The listing builds one solid part. Answer for the finished solid, in the listing's coordinates (mm). A direction names the side the tool comes from. Coordinates: 2 decimals unless noted, no trailing zeros. Loops run counter-clockwise (first coordinate to the right, second up) from the corner with the lowest first, then second, coordinate; pieces in that order, holes last. Notation, with made-up numbers: M 44,2.5 L 72,2.5 A8 ccw 72,8.5 Z; hole C 28,-29.75 d1. An arc over 180 degrees is marked long. Answer as a JSON object with one key per item and string values. Group by question number.
1. A cutting plane is placed at B-B on x = 8.5. Give the vertices of the cut face in (y, z).
2. Given pin 1 (6 mm diameter, centred on x = 1, y = -4.5, fed in from -Z); pin 2 (0.6 mm diameter, centred on y = -6.5, z = 1, fed in from +X); pin 3 (0.6 mm diameter, centred on x = -4.5, z = 1.5, fed in from -Y), each flat-ended and moving along its own axis, determine where each tip first touches the part or whether it passes through.
3. Straight lines are drawn through the part: L1, parallel to X at y = -7, z = 0.5; L2, parallel to Y at x = -4.5, z = 1.3; L3, parallel to X at y = 4.5, z = 1.05. For each, find the intervals that lie inside material, in ascending order.
4. For faces 1 (the face through (-4, -4, 1)), 2 (the face through (8, -4, 1)), 3 (the face through (2, 0, 0)), determine the directions among +Z, -Z, +X, -X, +Y, -Y from which every point of the face is accessible in a straight line to the end or side of a thin tool.
5. A cutting plane is placed at C-C on y = 5. Give the vertices of the cut face in (x, z).
6. A cutting plane is placed at A-A on z = 0.8. Give the vertices of the cut face in (x, y), and give its area (3 significant figures).
from build123d import *

# Parameters (mm, degrees)
BOSS_EXTRUDE1_DEPTH = 2


with BuildPart() as part:
    # Sketch1 → Boss-Extrude1 (new body)
    with BuildSketch(Plane.XY):
        with BuildLine():
            Line((5.533412898, -4), (10.466587102, -4))
            Line((10.466587102, -4), (10.466587102, 3))
            ThreePointArc((10.466587102, 3), (9.002121008, 6.535533906), (5.466587102, 8))
            Line((5.466587102, 8), (-6.466587102, 8))
            Line((-6.466587102, 8), (-6.466587102, -4))
            Line((-6.466587102, -4), (-2.466587102, -4))
            Line((-2.466587102, -4), (-2.466587102, -8))
            Line((-2.466587102, -8), (5.533412898, -8))
            Line((5.533412898, -8), (5.533412898, -4))
        make_face()
    extrude(amount=BOSS_EXTRUDE1_DEPTH)


solid = part.part
From the geometry:
{
 "1": {"outline": "M -4,0 L 6.97,0 L 6.97,2 L -4,2 Z"},
 "2": {"pin 1": "stops at z = 0", "pin 2": "stops at x = 5.53", "pin 3": "stops at y = -4"},
 "3": {"L1": "x = -2.47 to 5.53", "L2": "y = -4 to 8", "L3": "x = -6.47 to 10.24"},
 "4": {"face 1": "+Z, -Z, -X, -Y", "face 2": "+Z, -Z, +X, -Y", "face 3": "-Z, +X, -X, +Y, -Y"},
 "5": {"outline": "M -6.47,0 L 10.05,0 L 10.05,2 L -6.47,2 Z"},
 "6": {"outline": "M -6.47,-4 L -2.47,-4 L -2.47,-8 L 5.53,-8 L 5.53,-4 L 10.47,-4 L 10.47,3 A5 ccw 5.47,8 L -6.47,8 Z", "area": "230 mm²"}
}
